The listing builds one solid part. Answer for the finished solid, in the listing's coordinates (mm). Coordinates: 2 decimals unless noted, no trailing zeros. Write each loop counter-clockwise with the first axis right and the second up, starting at its lowest first coordinate (ties: lowest second). Pieces come first, ordered by that corner, then holes.
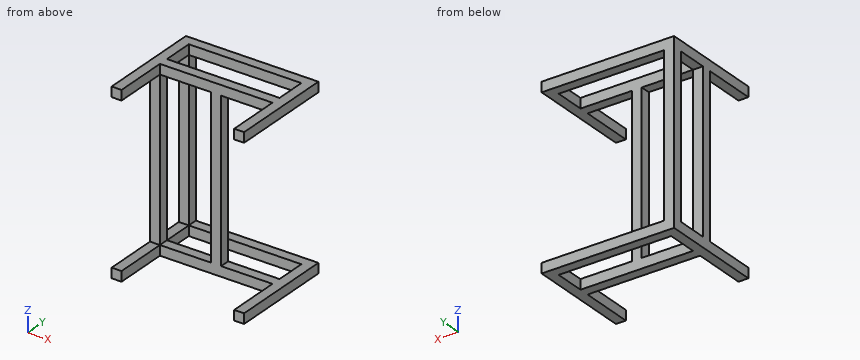
```python
from build123d import *

# Parameters (mm, degrees)
CROQUIS1_W              = 1016.2
CROQUIS1_H              = 1370
SALIENTE_EXTRUIR1_DEPTH = 800
CORTAR_EXTRUIR1_DEPTH   = 723.8
CROQUIS3_W              = 863.8
CROQUIS3_H              = 1217.6
CORTAR_EXTRUIR2_DEPTH   = 76.2
CROQUIS5_W              = 1217.6
CROQUIS5_H              = 76.2
SALIENTE_EXTRUIR2_DEPTH = 76.2
CROQUIS6_W              = 863.8
CROQUIS6_H              = 76.2
SALIENTE_EXTRUIR3_DEPTH = 76.2
CROQUIS7_W              = 1217.6
CROQUIS7_H              = 76.2
SALIENTE_EXTRUIR4_DEPTH = 76.2
CROQUIS8_W              = 863.8
CROQUIS8_H              = 76.2
SALIENTE_EXTRUIR5_DEPTH = 76.2
CROQUIS9_W              = 76.2
CROQUIS9_H              = 1217.6
CORTAR_EXTRUIR4_DEPTH   = 387.4
CROQUIS10_W             = 76.2
CROQUIS10_H             = 76.2
SALIENTE_EXTRUIR6_DEPTH = 1217.6


with BuildPart() as part:
    # Croquis1 → Saliente-Extruir1 (new body)
    with BuildSketch(Plane(origin=(0, 0, 0), x_dir=(1, 0, 0), z_dir=(0, 1, 0))):
        Rectangle(CROQUIS1_W, CROQUIS1_H)
    extrude(amount=SALIENTE_EXTRUIR1_DEPTH)

    # Croquis2 → Cortar-Extruir1 (cut)
    with BuildSketch(Plane.XZ):
        Polygon((431.9, 608.8), (431.9, 685), (-431.9, 685), (-431.9, 608.8), (-508.1, 608.8), (-508.1, -608.8), (-431.9, -608.8), (-431.9, -685), (431.9, -685), (431.9, -608.8), (508.1, -608.8), (508.1, 608.8), align=None)
    extrude(amount=-CORTAR_EXTRUIR1_DEPTH, mode=Mode.SUBTRACT)

    # Croquis3 → Cortar-Extruir2 (cut)
    with BuildSketch(Plane(origin=(0, 800, 0), x_dir=(1, 0, 0), z_dir=(0, 1, 0))):
        Rectangle(CROQUIS3_W, CROQUIS3_H)
    extrude(amount=-CORTAR_EXTRUIR2_DEPTH, mode=Mode.SUBTRACT)

    # Croquis5 → Saliente-Extruir2 (add)
    with BuildSketch(Plane.ZY.offset(508.1)):
        with Locations((0, 450.7)):
            Rectangle(CROQUIS5_W, CROQUIS5_H)
    extrude(amount=-SALIENTE_EXTRUIR2_DEPTH)

    # Croquis6 → Saliente-Extruir3 (add)
    with BuildSketch(Plane(origin=(0, 0, -685), x_dir=(-1, 0, 0), z_dir=(0, 0, -1))):
        with Locations((0, 450.7)):
            Rectangle(CROQUIS6_W, CROQUIS6_H)
    extrude(amount=-SALIENTE_EXTRUIR3_DEPTH)

    # Croquis7 → Saliente-Extruir4 (add)
    with BuildSketch(Plane(origin=(508.1, 0, 0), x_dir=(0, 0, -1), z_dir=(1, 0, 0))):
        with Locations((0, 450.7)):
            Rectangle(CROQUIS7_W, CROQUIS7_H)
    extrude(amount=-SALIENTE_EXTRUIR4_DEPTH)

    # Croquis8 → Saliente-Extruir5 (add)
    with BuildSketch(Plane.XY.offset(685)):
        with Locations((0, 450.7)):
            Rectangle(CROQUIS8_W, CROQUIS8_H)
    extrude(amount=-SALIENTE_EXTRUIR5_DEPTH)

    # Croquis9 → Cortar-Extruir4 (cut)
    with BuildSketch(Plane(origin=(0, 800, 0), x_dir=(1, 0, 0), z_dir=(0, 1, 0))):
        with Locations((470, 0)):
            Rectangle(CROQUIS9_W, CROQUIS9_H)
    extrude(amount=-CORTAR_EXTRUIR4_DEPTH, mode=Mode.SUBTRACT)

    # Croquis10 → Saliente-Extruir6 (add)
    with BuildSketch(Plane.XY.offset(-608.8)):
        with Locations((0, 450.7)):
            Rectangle(CROQUIS10_W, CROQUIS10_H)
    extrude(amount=SALIENTE_EXTRUIR6_DEPTH)


solid = part.part
```
(1) Section D-D, the plane y = 70 is taken. Write down the section's boundary in (x, z), plus the area to 3 significant figures.
(2) Section C-C, the plane y = 464 is taken. Write down the section's boundary in (x, z).
(3) Section A-A, the plane z = -336.5 is taken. Write down the section's boundary in (x, y), plus the area to 3 significant figures.
(4) Find the intervals of material crossed by probe 1 along X at (y, z) = (697.5, 625.5); probe 2 along Z at (x, y) = (-444.5, 85); probe 3 along Y at (x, z) = (-440, 427.5), in increasing order.
(5) Section B-B, the plane x = 124 is taken. Write down the section's boundary in (y, z).
Solution:
1. outline: (-508.1, -685) - (-431.9, -685) - (-431.9, -608.8) - (-508.1, -608.8) - close; (-508.1, 608.8) - (-431.9, 608.8) - (-431.9, 685) - (-508.1, 685) - close; (431.9, -685) - (508.1, -685) - (508.1, -608.8) - (431.9, -608.8) - close; (431.9, 608.8) - (508.1, 608.8) - (508.1, 685) - (431.9, 685) - close
1. area: 23,200 mm2
2. outline: (-508.1, -685) - (508.1, -685) - (508.1, -608.8) - (38.1, -608.8) - (38.1, 608.8) - (508.1, 608.8) - (508.1, 685) - (-508.1, 685) - close; hole (-431.9, -608.8) - (-38.1, -608.8) - (-38.1, 608.8) - (-431.9, 608.8) - close
3. outline: (-508.1, 412.6) - (-431.9, 412.6) - (-431.9, 488.8) - (-508.1, 488.8) - close; (-508.1, 723.8) - (-431.9, 723.8) - (-431.9, 800) - (-508.1, 800) - close; (-38.1, 412.6) - (38.1, 412.6) - (38.1, 488.8) - (-38.1, 488.8) - close
3. area: 17,400 mm2
4. probe 1: x = -508.1 to -431.9, 431.9 to 508.1
4. probe 2: z = -685 to -608.8, 608.8 to 685
4. probe 3: y = 412.6 to 488.8, 723.8 to 800
5. outline: (412.6, -685) - (488.8, -685) - (488.8, -608.8) - (412.6, -608.8) - close; (412.6, 608.8) - (488.8, 608.8) - (488.8, 685) - (412.6, 685) - close; (723.8, -685) - (800, -685) - (800, -608.8) - (723.8, -608.8) - close; (723.8, 608.8) - (800, 608.8) - (800, 685) - (723.8, 685) - close
